```python
from build123d import *

# Parameters (mm, degrees)
SKETCH_1_W          = 4
SKETCH_1_H          = 127.3
EXTRUDE_1_DEPTH     = 12.65
EXTRUDE_1_2_DEPTH   = 12.65
SKETCH_2_W          = 79.35
SKETCH_2_H          = 127.3
EXTRUDE_2_DEPTH     = 1.5
CUT_EXTRUDE_START   = -1.5
SKETCH_3_W          = 2.4
SKETCH_3_H          = 0.75
CUT_EXTRUDE_1_DEPTH = 133.588098372
SKETCH_4_W          = 71.35
SKETCH_4_H          = 1.5
EXTRUDE_3_DEPTH     = 12.65
SKETCH_6_W          = 7.5
SKETCH_6_H          = 9.8
EXTRUDE_5_DEPTH     = 9.6
SKETCH_7_R          = 2.05
CUT_EXTRUDE_2_DEPTH = 4.5
SKETCH_8_W          = 2.4
SKETCH_8_H          = 5.85
CUT_EXTRUDE_3_DEPTH = 8.55
SKETCH_10_W         = 3
SKETCH_10_H         = 5.95
EXTRUDE_6_DEPTH     = 3.95
SKETCH_11_W         = 40.5
SKETCH_11_H         = 5.95
EXTRUDE_7_DEPTH     = 0.35
FILLET_4_R          = 4
FILLET_5_R          = 2
SKETCH_12_W         = 41
SKETCH_12_H         = 4.65
CUT_EXTRUDE_4_DEPTH = 133.664871481
EXTRUDE_8_DEPTH     = 12.55
SKETCH_14_R         = 2.05
CUT_EXTRUDE_5_DEPTH = 7
SKETCH_15_W         = 7.5
SKETCH_15_H         = 7.5
EXTRUDE_9_DEPTH     = 5.55
SKETCH_16_R         = 2.05
CUT_EXTRUDE_6_DEPTH = 5


with BuildPart() as part:
    # Sketch 1 → Extrude 1 (new body)
    with BuildSketch(Plane(origin=(0, 0, 0), x_dir=(1, 0, 0), z_dir=(0, 1, 0))):
        with Locations((37.675, 0)):
            Rectangle(SKETCH_1_W, SKETCH_1_H)
    extrude(amount=EXTRUDE_1_DEPTH)



with BuildPart() as body_2:
    # Sketch 1 → Extrude 1 2 (new body)
    with BuildSketch(Plane(origin=(0, 0, 0), x_dir=(1, 0, 0), z_dir=(0, 1, 0))):
        with Locations((-37.675, 0)):
            Rectangle(SKETCH_1_W, SKETCH_1_H)
    extrude(amount=EXTRUDE_1_2_DEPTH)


with BuildPart() as part_1:
    add(part.part)

    add(body_2.part)  # Extrude 2 merges body 2
    # Sketch 2 → Extrude 2 (add)
    with BuildSketch(Plane(origin=(0, 12.65, 0), x_dir=(1, 0, 0), z_dir=(0, 1, 0))):
        Rectangle(SKETCH_2_W, SKETCH_2_H)
    extrude(amount=EXTRUDE_2_DEPTH)

    # Sketch 3 → Cut-Extrude 1 (cut, through all)
    with BuildSketch(Plane(origin=(0, 0, -63.65), x_dir=(-1, 0, 0), z_dir=(0, 0, -1)).offset(CUT_EXTRUDE_START)):
        with Locations((-36.875, 8.925)):
            Rectangle(SKETCH_3_W, SKETCH_3_H)
        with Locations((36.875, 8.925)):
            Rectangle(SKETCH_3_W, SKETCH_3_H)
    extrude(amount=-CUT_EXTRUDE_1_DEPTH, mode=Mode.SUBTRACT)

    # Sketch 4 → Extrude 3 (add)
    with BuildSketch(Plane.XZ.offset(-12.65)):
        with Locations((0, -62.9)):
            Rectangle(SKETCH_4_W, SKETCH_4_H)
    extrude(amount=EXTRUDE_3_DEPTH)

    # Sketch 6 → Extrude 5 (add)
    with BuildSketch(Plane.XZ.offset(-12.65)):
        with Locations((28.575, -57.25)):
            Rectangle(SKETCH_6_W, SKETCH_6_H)
    extrude(amount=EXTRUDE_5_DEPTH)

    # Sketch 7 → Cut-Extrude 2 (cut)
    with BuildSketch(Plane.XZ.offset(-3.05)):
        with Locations(Location((28.575, -56.1, 0), (0, 0, 270))):
            Circle(SKETCH_7_R)
    extrude(amount=-CUT_EXTRUDE_2_DEPTH, mode=Mode.SUBTRACT)

    # Sketch 8 → Cut-Extrude 3 (cut)
    with BuildSketch(Plane.XZ):
        with Locations((-36.875, 35.125)):
            Rectangle(SKETCH_8_W, SKETCH_8_H)
        with Locations((-36.875, -19.475)):
            Rectangle(SKETCH_8_W, SKETCH_8_H)
        with Locations((36.875, -19.475)):
            Rectangle(SKETCH_8_W, SKETCH_8_H)
        with Locations((36.875, 35.125)):
            Rectangle(SKETCH_8_W, SKETCH_8_H)
    extrude(amount=-CUT_EXTRUDE_3_DEPTH, mode=Mode.SUBTRACT)

    # Sketch 10 → Extrude 6 (add)
    with BuildSketch(Plane.XZ.offset(-12.65)):
        with Locations((-26.775, -54.725)):
            Rectangle(SKETCH_10_W, SKETCH_10_H)
        with Locations((16.725, -54.725)):
            Rectangle(SKETCH_10_W, SKETCH_10_H)
    extrude(amount=EXTRUDE_6_DEPTH)

    # Sketch 11 → Extrude 7 (add)
    with BuildSketch(Plane.XZ.offset(-12.65)):
        with Locations((-5.025, -54.725)):
            Rectangle(SKETCH_11_W, SKETCH_11_H)
    extrude(amount=EXTRUDE_7_DEPTH)

    # Fillet 4
    # the kernel refuses this fillet: 4 mm, written as the material it adds along each edge
    with BuildSketch(Plane(origin=(18.225, 12.65, -57.7), x_dir=(0, 0, -1), z_dir=(-1, 0, 0))) as fillet_4_piece_1_section:
        with BuildLine():
            CenterArc((FILLET_4_R, FILLET_4_R), FILLET_4_R, 180, 90)
            Line((0, FILLET_4_R), (0, 0))
            Line((0, 0), (FILLET_4_R, 0))
        make_face()
    fillet_4_piece_1 = extrude(amount=46.5, mode=Mode.PRIVATE)
    fillet_4_piece_1 = split(fillet_4_piece_1, bisect_by=Plane(origin=(15.225, 12.535953676, -59.259664423), z_dir=(1, 0, 0)), keep=Keep.TOP, mode=Mode.PRIVATE)
    fillet_4_piece_1 = split(fillet_4_piece_1, bisect_by=Plane(origin=(16.725, 12.3, -59.259664423), z_dir=(0, 1, 0)), keep=Keep.TOP, mode=Mode.PRIVATE)
    add(fillet_4_piece_1)
    with BuildSketch(Plane(origin=(18.225, 12.65, -57.7), x_dir=(0, 0, -1), z_dir=(-1, 0, 0))) as fillet_4_piece_2_section:
        with BuildLine():
            CenterArc((FILLET_4_R, FILLET_4_R), FILLET_4_R, 180, 90)
            Line((0, FILLET_4_R), (0, 0))
            Line((0, 0), (FILLET_4_R, 0))
        make_face()
    fillet_4_piece_2 = extrude(amount=46.5, mode=Mode.PRIVATE)
    fillet_4_piece_2 = split(fillet_4_piece_2, bisect_by=Plane(origin=(16.725, 8.7, -58.276150153), z_dir=(0, 1, 0)), keep=Keep.TOP, mode=Mode.PRIVATE)
    fillet_4_piece_2 = split(fillet_4_piece_2, bisect_by=Plane(origin=(15.225, 11.348610823, -58.276150153), z_dir=(1, 0, 0)), keep=Keep.TOP, mode=Mode.PRIVATE)
    fillet_4_piece_2 = split(fillet_4_piece_2, bisect_by=Plane(origin=(16.725, 12.3, -58.276150153), z_dir=(0, -1, 0)), keep=Keep.TOP, mode=Mode.PRIVATE)
    add(fillet_4_piece_2)
    with BuildSketch(Plane(origin=(18.225, 12.65, -57.7), x_dir=(0, 0, -1), z_dir=(-1, 0, 0))) as fillet_4_piece_3_section:
        with BuildLine():
            CenterArc((FILLET_4_R, FILLET_4_R), FILLET_4_R, 180, 90)
            Line((0, FILLET_4_R), (0, 0))
            Line((0, 0), (FILLET_4_R, 0))
        make_face()
    fillet_4_piece_3 = extrude(amount=46.5, mode=Mode.PRIVATE)
    fillet_4_piece_3 = split(fillet_4_piece_3, bisect_by=Plane(origin=(15.225, 12.535953676, -59.259664423), z_dir=(-1, 0, 0)), keep=Keep.TOP, mode=Mode.PRIVATE)
    fillet_4_piece_3 = split(fillet_4_piece_3, bisect_by=Plane(origin=(-5.025, 12.3, -59.259664423), z_dir=(0, 1, 0)), keep=Keep.TOP, mode=Mode.PRIVATE)
    fillet_4_piece_3 = split(fillet_4_piece_3, bisect_by=Plane(origin=(-25.275, 12.535953676, -59.259664423), z_dir=(1, 0, 0)), keep=Keep.TOP, mode=Mode.PRIVATE)
    add(fillet_4_piece_3)
    with BuildSketch(Plane(origin=(18.225, 12.65, -57.7), x_dir=(0, 0, -1), z_dir=(-1, 0, 0))) as fillet_4_piece_4_section:
        with BuildLine():
            CenterArc((FILLET_4_R, FILLET_4_R), FILLET_4_R, 180, 90)
            Line((0, FILLET_4_R), (0, 0))
            Line((0, 0), (FILLET_4_R, 0))
        make_face()
    fillet_4_piece_4 = extrude(amount=46.5, mode=Mode.PRIVATE)
    fillet_4_piece_4 = split(fillet_4_piece_4, bisect_by=Plane(origin=(-26.775, 12.3, -59.259664423), z_dir=(0, 1, 0)), keep=Keep.TOP, mode=Mode.PRIVATE)
    fillet_4_piece_4 = split(fillet_4_piece_4, bisect_by=Plane(origin=(-25.275, 12.535953676, -59.259664423), z_dir=(-1, 0, 0)), keep=Keep.TOP, mode=Mode.PRIVATE)
    add(fillet_4_piece_4)
    with BuildSketch(Plane(origin=(18.225, 12.65, -57.7), x_dir=(0, 0, -1), z_dir=(-1, 0, 0))) as fillet_4_piece_5_section:
        with BuildLine():
            CenterArc((FILLET_4_R, FILLET_4_R), FILLET_4_R, 180, 90)
            Line((0, FILLET_4_R), (0, 0))
            Line((0, 0), (FILLET_4_R, 0))
        make_face()
    fillet_4_piece_5 = extrude(amount=46.5, mode=Mode.PRIVATE)
    fillet_4_piece_5 = split(fillet_4_piece_5, bisect_by=Plane(origin=(-26.775, 8.7, -58.276150153), z_dir=(0, 1, 0)), keep=Keep.TOP, mode=Mode.PRIVATE)
    fillet_4_piece_5 = split(fillet_4_piece_5, bisect_by=Plane(origin=(-26.775, 12.3, -58.276150153), z_dir=(0, -1, 0)), keep=Keep.TOP, mode=Mode.PRIVATE)
    fillet_4_piece_5 = split(fillet_4_piece_5, bisect_by=Plane(origin=(-25.275, 11.348610823, -58.276150153), z_dir=(-1, 0, 0)), keep=Keep.TOP, mode=Mode.PRIVATE)
    add(fillet_4_piece_5)

    # Fillet 5
    fillet_5_edges = [part_1.edges().sort_by_distance(p)[0] for p in [
        (-26.775, 8.7, -57.700312512),
        (16.725, 8.7, -57.700312512),
    ]]
    fillet(fillet_5_edges, radius=FILLET_5_R)

    # Sketch 12 → Cut-Extrude 4 (cut, through all)
    with BuildSketch(Plane.XY.offset(-62.15)):
        with Locations((-5.025, 10.325)):
            Rectangle(SKETCH_12_W, SKETCH_12_H)
    extrude(amount=-CUT_EXTRUDE_4_DEPTH, mode=Mode.SUBTRACT)

    # Sketch 13 → Extrude 8 (add)
    with BuildSketch(Plane.XZ.offset(-12.65)):
        Polygon((-4.75, 60.9), (-4.75, 63.65), (4.75, 63.65), (4.75, 60.9), (4.75, 51.4), (-4.75, 51.4), align=None)
    extrude(amount=EXTRUDE_8_DEPTH)

    # Sketch 14 → Cut-Extrude 5 (cut)
    with BuildSketch(Plane.XZ.offset(-0.1)):
        with Locations(Location((0, 56.15, 0), (0, 0, 270))):
            Circle(SKETCH_14_R)
    extrude(amount=-CUT_EXTRUDE_5_DEPTH, mode=Mode.SUBTRACT)

    # Sketch 15 → Extrude 9 (add)
    with BuildSketch(Plane(origin=(0, 14.15, 0), x_dir=(1, 0, 0), z_dir=(0, 1, 0))):
        with Locations((33.89536, 55.44709)):
            Rectangle(SKETCH_15_W, SKETCH_15_H)
        with Locations((19.55046, -29.51121)):
            Rectangle(SKETCH_15_W, SKETCH_15_H)
    extrude(amount=EXTRUDE_9_DEPTH)

    # Sketch 16 → Cut-Extrude 6 (cut)
    with BuildSketch(Plane(origin=(0, 19.7, 0), x_dir=(1, 0, 0), z_dir=(0, 1, 0))):
        with Locations(Location((19.55046, -29.51121, 0), (0, 0, 270))):
            Circle(SKETCH_16_R)
        with Locations(Location((33.89536, 55.44709, 0), (0, 0, 270))):
            Circle(SKETCH_16_R)
    extrude(amount=-CUT_EXTRUDE_6_DEPTH, mode=Mode.SUBTRACT)


solid = part_1.part
```
Design review of the part built by this model. Coordinates are the model's own, in mm. A direction names the side the tool comes from. Coordinates: 2 decimals unless noted, no trailing zeros. Order: outer loops, then holes, each group sorted by start corner. A loop starts at its lowest first (then second) coordinate and runs counter-clockwise, first axis right, second up. Notation, with made-up numbers: M 26.25,44.25 L 80.25,44.25 A23 cw 80.25,60.25 Z; hole C 17.5,32 d6. An arc over 180 degrees is marked long. Answer as a JSON object with one key per item and string values. Group by question number.
1) Add section B-B, the plane x = 0. Write out the cut boundary in (y, z), then the cut area to 3 significant figures.
2) For pin 1 (0.8 mm diameter, centred on x = -6.5, z = -63.5, fed in from +Y); pin 2 (10 mm diameter, centred on x = -31, y = 15, fed in from +Z); pin 3 (5 mm diameter, centred on x = 20.5, y = 4, fed in from +Z); pin 4 (3.5 mm diameter, centred on x = 19.55, z = 29.51, fed in from +Y), all flat-tipped, find the tip position at first contact; note any pin that passes through.
3) Add section D-D, the plane y = 17.75. Write out the cut boundary in (x, z), then the cut area to 3 significant figures.
4) Wall thickness on L1, parallel to X at y = 5.55, z = -56.1 (3 decimals); L2, parallel to X at y = 2.25, z = 56.15 (3 decimals); L3, parallel to X at y = 12, z = 32.5 (3 decimals): over which ranges is each line inside the solid? List them lowest first.
5) Tool access review of faces 4 (the flat face through (-35.675, 11, 2)), 5 (the flat face through (0, 6, 51.4)), 6 (the flat face through (-38.075, 9, 10)), 7 (the flat face through (-37, 8.55, 51)), 8 (the flat face through (15.225, 10, -55)): name each direction out of +Z, -Z, +X, -X, +Y, -Y from which nothing blocks a thin tool from reaching the whole face with its end or side.
6) Mouldability with a two-part tool opening along Z and no side actions: class faces 1 (the cylindrical face through (27.8, 5.3, -58)), 2 (the flat face through (34, 14.7, -55)), 3 (the flat face through (15.8, 17, 30)) as pulls with the +Z half, pulls with the -Z half, needs draft (parallel to the pull), parting line crosses it, or undercut.
7) Add section C-C, the plane z = -41. Write out the cut boundary in (x, y) (3 decimals).
8) Add section A-A, the plane y = 5. Count the separate pieces of the cut face and the enclosed holes in it, then the cut area to 3 significant figures.
Computed values:
{
 "1": {"outline": "M 0,-63.65 L 8,-63.65 L 8,-62.15 L 0,-62.15 Z; M 0.1,51.4 L 12.65,51.4 L 12.65,-51.75 L 12.3,-51.75 L 12.3,-60.06 A4 cw 12.65,-61.7 L 12.65,-63.65 L 14.15,-63.65 L 14.15,63.65 L 0.1,63.65 L 0.1,58.2 L 7.1,58.2 L 7.1,54.1 L 0.1,54.1 Z", "area": "331 mm^2"},
 "2": {"pin 1": "stops at y = 14.15", "pin 2": "stops at z = 63.65", "pin 3": "stops at z = -62.15", "pin 4": "stops at y = 14.7"},
 "3": {"outline": "M 15.8,25.76 L 23.3,25.76 L 23.3,33.26 L 15.8,33.26 Z; M 30.15,-59.2 L 37.65,-59.2 L 37.65,-51.7 L 30.15,-51.7 Z; hole C 19.55,29.51 d4.1; hole C 33.9,-55.45 d4.1", "area": "86.1 mm^2"},
 "4": {"L1": "x = -39.675 to -35.675, 24.825 to 26.525, 30.625 to 32.325, 35.675 to 39.675", "L2": "x = -39.675 to -35.675, -4.75 to -2.05, 2.05 to 4.75, 35.675 to 39.675", "L3": "x = -39.675 to -35.675, 35.675 to 39.675"},
 "5": {"face 4": "+Z, -Y", "face 5": "-Y", "face 6": "none", "face 7": "+Z", "face 8": "+Z, -Z, -Y"},
 "6": {"face 1": "undercut", "face 2": "undercut", "face 3": "needs draft"},
 "7": {"outline": "M -39.675,0 L -35.675,0 L -35.675,8.55 L -38.075,8.55 L -38.075,9.3 L -35.675,9.3 L -35.675,12.65 L 35.675,12.65 L 35.675,9.3 L 38.075,9.3 L 38.075,8.55 L 35.675,8.55 L 35.675,0 L 39.675,0 L 39.675,14.15 L -39.675,14.15 Z"},
 "8": {"separate pieces": "2", "enclosed holes": "2", "area": "1,230 mm^2"}
}
